Autodesk Inventor part; units mm, degrees
ref_plane "YZ Plane" through (0, 0, 0) normal (1, 0, 0) x (0, 1, 0)
ref_plane "XZ Plane" through (0, 0, 0) normal (0, 1, 0) x (-1, 0, 0)
ref_plane "XY Plane" through (0, 0, 0) normal (0, 0, 1) x (1, 0, 0)
sketch "Sketch1" plane through (0, 0, 0) normal (0, 0, 1) x (1, 0, 0)
  line L0 (-34.86, 0) -> (34.86, 0) construction
  line L1 (0, -34.86) -> (0, 34.86) construction
  line L2 (0, 0) -> (11.1575, 11.1575) construction
  line L3 (0, 0) -> (15.7791, 0) construction
  line L4 (0, 24.9) -> (16.8009, 24.9)
  line L5 (16.8009, 24.9) -> (16.8009, 21.2415)
  line L6 (16.8009, 21.2415) -> (19.0212, 19.0212)
  line L7 (24.9, 0) -> (24.9, 16.8009)
  line L8 (24.9, 16.8009) -> (21.2415, 16.8009)
  line L9 (21.2415, 16.8009) -> (19.0212, 19.0212)
  line L10 (0, -24.9) -> (16.8009, -24.9)
  line L11 (16.8009, -24.9) -> (16.8009, -21.2415)
  line L12 (16.8009, -21.2415) -> (19.0212, -19.0212)
  line L13 (24.9, 0) -> (24.9, -16.8009)
  line L14 (24.9, -16.8009) -> (21.2415, -16.8009)
  line L15 (21.2415, -16.8009) -> (19.0212, -19.0212)
  line L16 (0, 24.9) -> (-16.8009, 24.9)
  line L17 (-16.8009, 24.9) -> (-16.8009, 21.2415)
  line L18 (-16.8009, 21.2415) -> (-19.0212, 19.0212)
  line L19 (-24.9, 16.8009) -> (-21.2415, 16.8009)
  line L20 (-21.2415, 16.8009) -> (-19.0212, 19.0212)
  line L21 (0, -24.9) -> (-16.8009, -24.9)
  line L22 (-16.8009, -24.9) -> (-16.8009, -21.2415)
  line L23 (-16.8009, -21.2415) -> (-19.0212, -19.0212)
  line L24 (-21.2415, -16.8009) -> (-19.0212, -19.0212)
  line L25 (-24.9, -16.8009) -> (-21.2415, -16.8009)
  line L26 (-24.9, 0) -> (-24.9, -16.8009)
  line L27 (-24.9, 0) -> (-24.9, 16.8009)
  circle A0 centre (0, 0) radius 12.5
  dimension "d0" = 45
  dimension "d2" = 24.9
  dimension "d3" = 3.14
  dimension "d4" = 26.9
  dimension "d5" = 25
extrude "Extrusion1" add sketch "Sketch1" along normal blind 5
sketch "Sketch3" plane through (0, 0, 0) normal (0, 0, -1) x (-1, 0, 0)
  circle A0 centre (0, 0) radius 12.5
extrude "Extrusion3" add sketch "Sketch3" against normal blind 3
sketch "Sketch4" plane through (0, 0, 3) normal (0, 0, 1) x (1, 0, 0)
  circle A0 centre (0, 0) radius 12.5
  arc A1 (-2.4955, 9.5466) -> (2.5955, 9.5466) centre (0.05, 10.5454) ccw
  arc A2 (-2.4955, 9.5466) -> (-3.0679, 9.7469) centre (-2.8679, 9.4005) ccw
  line L0 (-3.0679, 9.7469) -> (-6.8321, 7.5736)
  arc A3 (-6.8321, 7.5736) -> (-6.9449, 6.9778) centre (-6.6321, 7.2272) ccw
  arc A4 (-9.4904, 2.5688) -> (-6.9449, 6.9778) centre (-9.0826, 5.2727) ccw
  arc A5 (2.5955, -9.5466) -> (-2.4955, -9.5466) centre (0.05, -10.5454) ccw
  arc A6 (2.5955, -9.5466) -> (3.1679, -9.7469) centre (2.9679, -9.4005) ccw
  line L1 (3.1679, -9.7469) -> (6.9321, -7.5736)
  arc A7 (6.9321, -7.5736) -> (7.0449, -6.9778) centre (6.7321, -7.2272) ccw
  arc A8 (9.5904, -2.5688) -> (7.0449, -6.9778) centre (9.1826, -5.2727) ccw
  line L2 (5.3229, -1.93) -> (5.3229, -1.58)
  line L3 (5.3229, -1.58) -> (5.9268, -1.58)
  line L4 (6.2768, -2.56) -> (5.9268, -2.56)
  line L5 (5.9268, -2.56) -> (5.9268, -1.93)
  line L6 (5.9268, -1.93) -> (5.3229, -1.93)
  circle A9 centre (0.05, 0) radius 3.3699
  line L7 (1.2704, -6.4878) -> (4.6724, -4.4373)
  line L8 (4.6724, -4.4373) -> (5.9738, -6.5964)
  line L9 (5.9738, -6.5964) -> (2.5718, -8.647)
  line L10 (2.5718, -8.647) -> (1.2704, -6.4878)
  line L11 (-2.4718, 8.647) -> (-1.1704, 6.4878)
  line L12 (-1.1704, 6.4878) -> (-4.5724, 4.4373)
  line L13 (-4.5724, 4.4373) -> (-5.8738, 6.5964)
  line L14 (-5.8738, 6.5964) -> (-2.4718, 8.647)
  arc A10 (-3.5679, -10.6129) -> (-1.5646, -9.9119) centre (-2.8679, -9.4005) ccw
  line L15 (-3.5679, -10.6129) -> (-7.3321, -8.4396)
  arc A11 (-7.7266, -6.3542) -> (-7.3321, -8.4396) centre (-6.6321, -7.2272) ccw
  arc A12 (-7.7266, -6.3542) -> (-9.3412, -3.5577) centre (-9.0826, -5.2727) ccw
  arc A13 (-10.95, -2.1733) -> (-9.3412, -3.5577) centre (-9.55, -2.1733) ccw
  line L16 (-10.95, -2.1733) -> (-10.95, 2.1733)
  arc A14 (-9.3412, 3.5577) -> (-10.95, 2.1733) centre (-9.55, 2.1733) ccw
  arc A15 (-9.3412, 3.5577) -> (-7.7266, 6.3542) centre (-9.0826, 5.2727) ccw
  arc A16 (-7.3321, 8.4396) -> (-7.7266, 6.3542) centre (-6.6321, 7.2272) ccw
  line L17 (-7.3321, 8.4396) -> (-3.5679, 10.6129)
  arc A17 (-1.5646, 9.9119) -> (-3.5679, 10.6129) centre (-2.8679, 9.4005) ccw
  arc A18 (-1.5646, 9.9119) -> (1.6646, 9.9119) centre (0.05, 10.5454) ccw
  arc A19 (3.6679, 10.6129) -> (1.6646, 9.9119) centre (2.9679, 9.4005) ccw
  line L18 (3.6679, 10.6129) -> (7.4321, 8.4396)
  arc A20 (7.8266, 6.3542) -> (7.4321, 8.4396) centre (6.7321, 7.2272) ccw
  arc A21 (7.8266, 6.3542) -> (9.4412, 3.5577) centre (9.1826, 5.2727) ccw
  arc A22 (11.05, 2.1733) -> (9.4412, 3.5577) centre (9.65, 2.1733) ccw
  line L19 (11.05, 2.1733) -> (11.05, -2.1733)
  arc A23 (9.4412, -3.5577) -> (11.05, -2.1733) centre (9.65, -2.1733) ccw
  arc A24 (9.4412, -3.5577) -> (7.8266, -6.3542) centre (9.1826, -5.2727) ccw
  arc A25 (7.4321, -8.4396) -> (7.8266, -6.3542) centre (6.7321, -7.2272) ccw
  line L20 (7.4321, -8.4396) -> (3.6679, -10.6129)
  arc A26 (1.6646, -9.9119) -> (3.6679, -10.6129) centre (2.9679, -9.4005) ccw
  arc A27 (1.6646, -9.9119) -> (-1.5646, -9.9119) centre (0.05, -10.5454) ccw
  arc A28 (7.0449, 6.9778) -> (6.9321, 7.5736) centre (6.7321, 7.2272) ccw
  line L21 (6.9321, 7.5736) -> (3.1679, 9.7469)
  arc A29 (3.1679, 9.7469) -> (2.5955, 9.5466) centre (2.9679, 9.4005) ccw
  arc A30 (-9.4904, 2.5688) -> (-9.95, 2.1733) centre (-9.55, 2.1733) ccw
  line L22 (-9.95, 2.1733) -> (-9.95, -2.1733)
  arc A31 (-9.95, -2.1733) -> (-9.4904, -2.5688) centre (-9.55, -2.1733) ccw
  arc A32 (-6.9449, -6.9778) -> (-9.4904, -2.5688) centre (-9.0826, -5.2727) ccw
  arc A33 (-6.9449, -6.9778) -> (-6.8321, -7.5736) centre (-6.6321, -7.2272) ccw
  line L23 (-6.8321, -7.5736) -> (-3.0679, -9.7469)
  arc A34 (-3.0679, -9.7469) -> (-2.4955, -9.5466) centre (-2.8679, -9.4005) ccw
  arc A35 (9.5904, -2.5688) -> (10.05, -2.1733) centre (9.65, -2.1733) ccw
  line L24 (10.05, -2.1733) -> (10.05, 2.1733)
  arc A36 (10.05, 2.1733) -> (9.5904, 2.5688) centre (9.65, 2.1733) ccw
  arc A37 (7.0449, 6.9778) -> (9.5904, 2.5688) centre (9.1826, 5.2727) ccw
  line L25 (5.9268, -1.58) -> (5.9268, -0.96)
  line L26 (5.9268, -0.96) -> (6.2768, -0.96)
  line L27 (6.2768, -0.96) -> (6.2768, -1.58)
  line L28 (6.2768, -1.58) -> (6.9229, -1.58)
  line L29 (6.9229, -1.58) -> (6.9229, -1.93)
  line L30 (6.9229, -1.93) -> (6.2768, -1.93)
  line L31 (6.2768, -1.93) -> (6.2768, -2.56)
  line L32 (-1.1704, -6.4878) -> (-2.4718, -8.647)
  line L33 (-2.4718, -8.647) -> (-5.8738, -6.5964)
  line L34 (-5.8738, -6.5964) -> (-4.5724, -4.4373)
  line L35 (-4.5724, -4.4373) -> (-1.1704, -6.4878)
  line L36 (5.9738, 6.5964) -> (4.6724, 4.4373)
  line L37 (4.6724, 4.4373) -> (1.2704, 6.4878)
  line L38 (1.2704, 6.4878) -> (2.5718, 8.647)
  line L39 (2.5718, 8.647) -> (5.9738, 6.5964)
  line L40 (-8.6062, -2.0991) -> (-8.6062, 0.1709)
  line L41 (-8.6062, 0.1709) -> (-5.5375, 0.1709)
  line L42 (-5.5375, 0.1709) -> (-5.5375, -2.0991)
  line L43 (-5.5375, -2.0991) -> (-8.6062, -2.0991)
  line L44 (-6.8834, 0.8144) -> (-6.8834, 2.4144)
  line L45 (-6.8834, 2.4144) -> (-6.5334, 2.4144)
  line L46 (-6.5334, 2.4144) -> (-6.5334, 0.8144)
  line L47 (-6.5334, 0.8144) -> (-6.8834, 0.8144)
  line L48 (5.5596, -0.1311) -> (5.5596, 2.208)
  line L49 (5.5596, 2.208) -> (8.9002, 2.208)
  line L50 (8.9002, 2.208) -> (8.9002, -0.1311)
  line L51 (8.9002, -0.1311) -> (5.5596, -0.1311)
  point P0 (0.05, 10.5454)
  point P1 (-9.0826, 5.2727)
  point P2 (0.05, -10.5454)
  point P3 (9.1826, -5.2727)
  dimension "d15" = 1
extrude "Extrusion4" add sketch "Sketch4" along normal up to surface (2 mm away) contours A0
sketch "Skizze5" plane through (0, 0, 5) normal (0, 0, 1) x (1, 0, 0)
  line L0 (-7.3321, -8.4396) -> (-3.5679, -10.6129) construction
  arc A0 (-7.7266, -6.3542) -> (-7.3321, -8.4396) centre (-6.6321, -7.2272) ccw construction
  arc A1 (-7.7266, -6.3542) -> (-9.3412, -3.5577) centre (-9.0826, -5.2727) ccw construction
  arc A2 (-10.95, -2.1733) -> (-9.3412, -3.5577) centre (-9.55, -2.1733) ccw construction
  line L1 (-10.95, 2.1733) -> (-10.95, -2.1733) construction
  arc A3 (-9.3412, 3.5577) -> (-10.95, 2.1733) centre (-9.55, 2.1733) ccw construction
  arc A4 (-9.3412, 3.5577) -> (-7.7266, 6.3542) centre (-9.0826, 5.2727) ccw construction
  arc A5 (-7.3321, 8.4396) -> (-7.7266, 6.3542) centre (-6.6321, 7.2272) ccw construction
  line L2 (-3.5679, 10.6129) -> (-7.3321, 8.4396) construction
  arc A6 (-1.5646, 9.9119) -> (-3.5679, 10.6129) centre (-2.8679, 9.4005) ccw construction
  arc A7 (-1.5646, 9.9119) -> (1.6646, 9.9119) centre (0.05, 10.5454) ccw construction
  arc A8 (3.6679, 10.6129) -> (1.6646, 9.9119) centre (2.9679, 9.4005) ccw construction
  line L3 (7.4321, 8.4396) -> (3.6679, 10.6129) construction
  arc A9 (7.8266, 6.3542) -> (7.4321, 8.4396) centre (6.7321, 7.2272) ccw construction
  arc A10 (7.8266, 6.3542) -> (9.4412, 3.5577) centre (9.1826, 5.2727) ccw construction
  arc A11 (11.05, 2.1733) -> (9.4412, 3.5577) centre (9.65, 2.1733) ccw construction
  line L4 (11.05, -2.1733) -> (11.05, 2.1733) construction
  arc A12 (9.4412, -3.5577) -> (11.05, -2.1733) centre (9.65, -2.1733) ccw construction
  arc A13 (9.4412, -3.5577) -> (7.8266, -6.3542) centre (9.1826, -5.2727) ccw construction
  arc A14 (7.4321, -8.4396) -> (7.8266, -6.3542) centre (6.7321, -7.2272) ccw construction
  line L5 (3.6679, -10.6129) -> (7.4321, -8.4396) construction
  arc A15 (1.6646, -9.9119) -> (3.6679, -10.6129) centre (2.9679, -9.4005) ccw construction
  arc A16 (1.6646, -9.9119) -> (-1.5646, -9.9119) centre (0.05, -10.5454) ccw construction
  arc A17 (-3.5679, -10.6129) -> (-1.5646, -9.9119) centre (-2.8679, -9.4005) ccw construction
  line L6 (16.8009, 24.9) -> (-16.8009, 24.9) construction
  line L7 (-16.8009, 24.9) -> (-16.8009, 21.2415)
  line L8 (-16.8009, 21.2415) -> (-21.2415, 16.8009)
  line L9 (-21.2415, 16.8009) -> (-24.9, 16.8009)
  line L10 (-24.9, 16.8009) -> (-24.9, -16.8009) construction
  line L11 (-24.9, -16.8009) -> (-21.2415, -16.8009)
  line L12 (-21.2415, -16.8009) -> (-16.8009, -21.2415)
  line L13 (-16.8009, -21.2415) -> (-16.8009, -24.9)
  line L14 (-16.8009, -24.9) -> (16.8009, -24.9) construction
  line L15 (16.8009, -24.9) -> (16.8009, -21.2415)
  line L16 (16.8009, -21.2415) -> (21.2415, -16.8009)
  line L17 (21.2415, -16.8009) -> (24.9, -16.8009)
  line L18 (24.9, -16.8009) -> (24.9, 16.8009) construction
  line L19 (24.9, 16.8009) -> (21.2415, 16.8009)
  line L20 (21.2415, 16.8009) -> (16.8009, 21.2415)
  line L21 (16.8009, 21.2415) -> (16.8009, 24.9)
  line L22 (-17.0009, 25.1) -> (17.0009, 25.1) construction
  line L23 (17.0009, 25.1) -> (17.0009, 21.3243)
  line L24 (17.0009, 21.3243) -> (21.3243, 17.0009)
  line L25 (21.3243, 17.0009) -> (25.1, 17.0009)
  line L26 (25.1, 17.0009) -> (25.1, -17.0009) construction
  line L27 (25.1, -17.0009) -> (21.3243, -17.0009)
  line L28 (21.3243, -17.0009) -> (17.0009, -21.3243)
  line L29 (17.0009, -21.3243) -> (17.0009, -25.1)
  line L30 (17.0009, -25.1) -> (-17.0009, -25.1) construction
  line L31 (-17.0009, -25.1) -> (-17.0009, -21.3243)
  line L32 (-17.0009, -21.3243) -> (-21.3243, -17.0009)
  line L33 (-21.3243, -17.0009) -> (-25.1, -17.0009)
  line L34 (-25.1, -17.0009) -> (-25.1, 17.0009) construction
  line L35 (-25.1, 17.0009) -> (-21.3243, 17.0009)
  line L36 (-21.3243, 17.0009) -> (-17.0009, 21.3243)
  line L37 (-17.0009, 21.3243) -> (-17.0009, 25.1)
  line L38 (-21.2415, 16.8009) -> (-24.9, 16.8009)
  line L39 (-24.9, 16.8009) -> (-24.9, 17.0009)
  line L40 (-16.8009, 24.9) -> (-17.0009, 24.9)
  line L41 (16.8009, 24.9) -> (-16.8009, 24.9)
  line L42 (16.8009, 24.9) -> (17.0009, 24.9)
  line L43 (24.9, 16.8009) -> (21.2415, 16.8009)
  line L44 (24.9, 16.8009) -> (24.9, 17.0009)
  line L45 (24.9, -16.8009) -> (24.9, -17.0009)
  line L46 (16.8009, -24.9) -> (16.8009, -21.2415)
  line L47 (16.8009, -24.9) -> (17.0009, -24.9)
  line L48 (-16.8009, -21.2415) -> (-16.8009, -24.9)
  line L49 (-16.8009, -24.9) -> (-17.0009, -24.9)
  line L50 (-24.9, -16.8009) -> (-24.9, -17.0009)
  point P0 (0, 0)
  dimension "d18" = 0.2
extrude "IM_offset" add sketch "Skizze5" against normal up to surface (5 mm away)
properties part number "20_Cube_insert_Sample_holder"
The listing builds one solid part. Answer for the finished solid, in the listing's coordinates (mm). A direction names the side the tool comes from. Coordinates: 2 decimals unless noted, no trailing zeros. Loops run counter-clockwise (first coordinate to the right, second up) from the corner with the lowest first, then second, coordinate; pieces in that order, holes last. Notation, with made-up numbers: (34.25, -37.75) -> (83.25, -37.75) arc R18 ccw to (83.25, -15.75) -> close; hole circle Ø5 at (-22.5, 72). An arc over 180 degrees is marked (long way). Answer in a Markdown table with one row per item. Add a question column.
1. For faces 1 (the flat face through (0, 0, 3)), 2 (the flat face through (17.001, 23, 3)), 3 (the flat face through (-19.132, -19.193, 2.535)), determine the directions among +Z, -Z, +X, -X, +Y, -Y from which every point of the face is accessible in a straight line to the end or side of a thin tool.
2. The part is cut by section B-B, the plane y = 7. Write down the section's boundary in (x, z), then the cut area to 3 significant figures.
3. Determine the mould class of faces 4 (the flat face through (17.001, -23, 3)), 5 (the flat face through (-19.193, 19.132, 2.535)), 6 (the flat face through (0, 0, 0)), 7 (the cylindrical face through (2.521, -10.727, 3.986)) for opening direction X: +X half, -X half, draft (parallel to the pull), parting line (faces both ways), or undercut.
4. Consider line 1 (Y direction, x = 9, z = 3.55); line 2 (X direction, y = -10, z = 3.75); line 3 (X direction, y = -4.5, z = 3.1). Determine where each line is inside the solid, lowest interval first. Write a range as [from, to].
5. The part is cut by section A-A, the plane z = 2.1. Write down the section's boundary in (x, y).
6. The part is cut by section C-C, the plane x = 2.5. Write down the section's boundary in (y, z), then the cut area to 3 significant figures.
7. Flat-ended cylindrical pins translate along their axes: P1, Ø1.5, axis at x = 19.5, z = 4, coming from the -Y side; P2, Ø3, axis at x = -22.5, z = 2, coming from the +Y side; P3, Ø1.1, axis at x = 23, z = 1.5, coming from the -Y side. Find the tip coordinate at first contact, or state that the pin passes through.
8. The part is cut by section D-D, the plane y = 19. Write down the section's boundary in (x, z), then the cut area to 3 significant figures.
Answer below:
| question | item | result |
|---|---|---|
| 1 | face 1 | +Z |
| 1 | face 2 | +Z, -Z, +X, +Y |
| 1 | face 3 | +Z, -Z, -X, -Y |
| 2 | outline | (-24.9, 0) -> (24.9, 0) -> (24.9, 5) -> (8.11, 5) -> (8.11, 3) -> (-8.01, 3) -> (-8.01, 5) -> (-24.9, 5) -> close |
| 2 | area | 217 mm2 |
| 3 | face 4 | +X half |
| 3 | face 5 | -X half |
| 3 | face 6 | draft |
| 3 | face 7 | undercut |
| 4 | line 1 | [-24.9, -3.55], [3.55, 24.9] |
| 4 | line 2 | [-24.9, -4.63], [-1.6, 1.7], [4.73, 24.9] |
| 4 | line 3 | [-24.9, -7.53], [7.63, 24.9] |
| 5 | outline | (-24.9, -17) -> (-21.32, -17) -> (-17, -21.32) -> (-17, -24.9) -> (17, -24.9) -> (17, -21.32) -> (21.32, -17) -> (24.9, -17) -> (24.9, 17) -> (21.32, 17) -> (17, 21.32) -> (17, 24.9) -> (-17, 24.9) -> (-17, 21.32) -> (-21.32, 17) -> (-24.9, 17) -> close |
| 6 | outline | (-24.9, 0) -> (24.9, 0) -> (24.9, 5) -> (10.72, 5) -> (10.72, 3) -> (-10.72, 3) -> (-10.72, 5) -> (-24.9, 5) -> close |
| 6 | area | 206 mm2 |
| 7 | P1 | y = -19.58 |
| 7 | P2 | y = 17.33 |
| 7 | P3 | y = -17 |
| 8 | outline | (-19.33, 0) -> (19.33, 0) -> (19.33, 5) -> (-19.33, 5) -> close |
| 8 | area | 193 mm2 |
